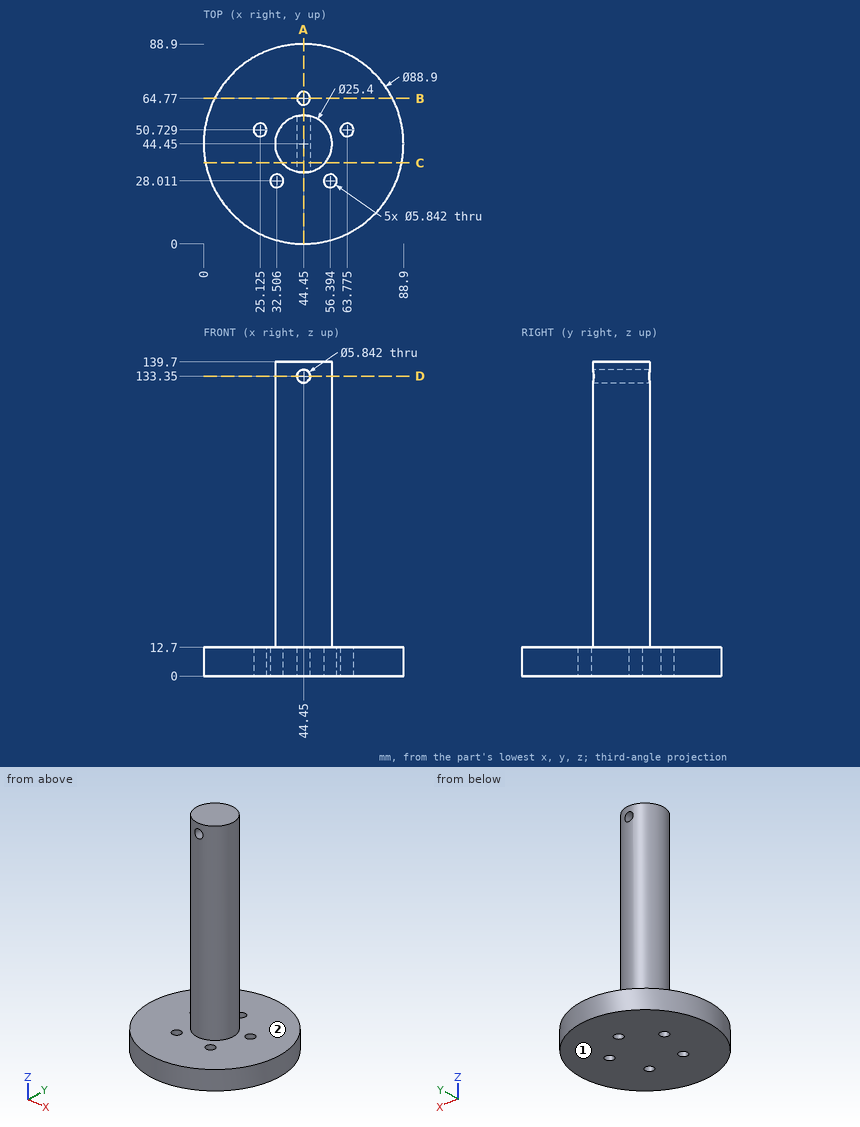
Design review of the part shown in the three views and the two pictorial views. Dimensions are in mm from the part's minimum x, y and z. A direction names the side the tool comes from. Give positions to 0.01 mm unless a question says otherwise; leave off trailing zeros. Write each loop counter-clockwise with the first axis right and the second up, starting at its lowest first coordinate (ties: lowest second). Pieces come first, ordered by that corner, then holes. Notation, with made-up numbers: M 36.5,-4 L 87.5,-4 A14 cw 87.5,6 Z; hole C 71.5,-15 d10. An arc over 180 degrees is marked long. Return JSON: item names as keys, results as strings. Group by question number.
Item 1: Wall thickness on line 1 along Z through (x, y) = (44.5, 38); line 2 along Z through (x, y) = (61, 54.5); line 3 along X through (y, z) = (42, 133): over which ranges is each line inside the solid? List them lowest first.
Item 2: Tool access review of the marked faces 1 and 2: name each direction out of +Z, -Z, +X, -X, +Y, -Y from which nothing blocks a thin tool from reaching the whole face with its end or side.
Item 3: Take a section at D-D (z = 133.35). Give the boundary of the cut face in (x, y).
Item 4: Take a section at A-A (x = 44.45). Give the boundary of the cut face in (y, z), plus the area to 3 significant figures.
Item 5: Take a section at B-B (y = 64.77). Give the boundary of the cut face in (x, z), plus the area to 3 significant figures.
Item 6: Clearance check with flat-ended pins moving along their axes: pin 1 Ø2 at (x, y) = (24, 61.5) entering from -Z; pin 2 Ø5.5 at (x, z) = (44.45, 133.35) entering from -Y. State where each tip first meets the part, or that it passes through.
Item 7: Take a section at C-C (y = 36). Give the boundary of the cut face in (x, z), plus the area to 3 significant figures.
Return value:
{
 "1": {"line 1": "z = 0 to 130.43, 136.27 to 139.7", "line 2": "z = 0 to 12.7", "line 3": "x = 31.99 to 41.55, 47.35 to 56.91"},
 "2": {"face 1": "-Z, +X, -X, +Y, -Y", "face 2": "+Z"},
 "3": {"outline": "M 41.53,32.09 L 41.53,56.81 A12.7 ccw Z; M 47.37,32.09 A12.7 ccw 47.37,56.81 Z"},
 "4": {"outline": "M 0,0 L 61.85,0 L 61.85,12.7 L 57.15,12.7 L 57.15,130.43 L 31.75,130.43 L 31.75,12.7 L 0,12.7 Z; M 31.75,136.27 L 57.15,136.27 L 57.15,139.7 L 31.75,139.7 Z; M 67.69,0 L 88.9,0 L 88.9,12.7 L 67.69,12.7 Z", "area": "4,130 mm2"},
 "5": {"outline": "M 4.92,0 L 41.53,0 L 41.53,12.7 L 4.92,12.7 Z; M 47.37,0 L 83.98,0 L 83.98,12.7 L 47.37,12.7 Z", "area": "930 mm2"},
 "6": {"pin 1": "stops at z = 0", "pin 2": "passes through"},
 "7": {"outline": "M 0.81,0 L 88.09,0 L 88.09,12.7 L 53.93,12.7 L 53.93,139.7 L 34.97,139.7 L 34.97,12.7 L 0.81,12.7 Z; hole C 44.45,133.35 d5.84", "area": "3,490 mm2"}
}
